Verification items for the finished model (mm, model axes). Round coordinates to 2 decimals unless told otherwise and drop trailing zeros. Loops run counter-clockwise (first coordinate to the right, second up) from the corner with the lowest first, then second, coordinate; pieces in that order, holes last. Notation, with made-up numbers: (86, -15) -> (110, -15) arc R30 ccw to (110, 9) -> close; hole circle Ø7 at (7.5, -3). An arc over 180 degrees is marked (long way). Use a Markdown table: item, result. Add a question column.
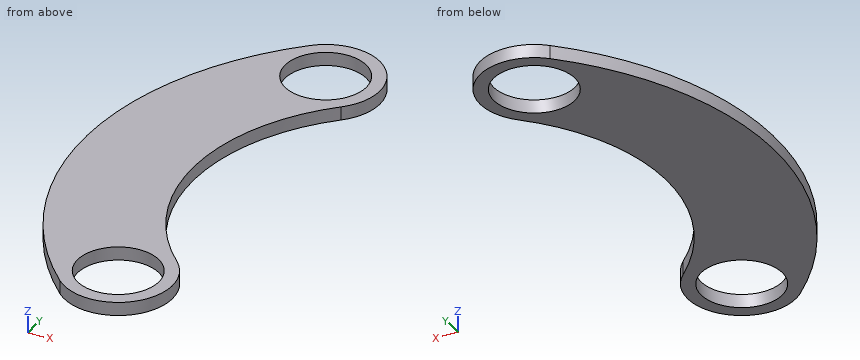
```python
from build123d import *

# Parameters (mm, degrees)
ESQUISSE1_R               = 3
T_LE_DE_BASE_PLI_E1_DEPTH = 1


# Sheet-metal steps are written as plain solids
with BuildPart() as part:
    # Esquisse1 → Tôle de base pliée1 (new body)
    with BuildSketch(Plane.XY):
        with BuildLine():
            ThreePointArc((-57.239284083, -19.336263861), (-64.490656247, -36.242246604), (-57.218655547, -53.139366375))
            ThreePointArc((-57.218655547, -53.139366375), (-51.563834313, -52.987719377), (-51.715481312, -47.332898143))
            ThreePointArc((-51.715481312, -47.332898143), (-56.490657737, -36.237364559), (-51.729027089, -25.136011084))
            ThreePointArc((-51.729027089, -25.136011084), (-51.584281974, -19.481008975), (-57.239284083, -19.336263861))
        make_face()
        with Locations((-54.484155586, -22.236137473)):
            Circle(ESQUISSE1_R, mode=Mode.SUBTRACT)
        with Locations((-54.467068429, -50.236132259)):
            Circle(ESQUISSE1_R, mode=Mode.SUBTRACT)
    extrude(amount=-T_LE_DE_BASE_PLI_E1_DEPTH)


solid = part.part
```
1) Sectioned sample at B-B on y = -49. Enter the section's corners in (x, z).
2) Sectioned sample at D-D on y = -40.5. Enter the section's corners in (x, z), then the cut area to 3 significant figures.
3) Sectioned sample at C-C on z = -0.6. Enter the section's corners in (x, y), then the cut area to 3 significant figures.
4) Go/stop test with a flat-tipped pin: pin 1 (5.5 mm diameter, centred on x = -54.48, y = -22.24, fed in from -Z). Record where the tip stops, or that it passes through.
5) Thickness scan on line 1 (Y direction, x = -54.5, z = -0.9); line 2 (Y direction, x = -52.5, z = -0.8); line 3 (Y direction, x = -51, z = -0.7). Record the ranges inside material, lowest first.
6) Sectioned sample at A-A on x = -53.75. Enter the section's corners in (y, z), then the cut area to 3 significant figures.
Geometry results:
| question | item | result |
|---|---|---|
| 1 | outline | (-60.68, -1) -> (-57.2, -1) -> (-57.2, 0) -> (-60.68, 0) -> close; (-51.73, -1) -> (-50.66, -1) -> (-50.66, 0) -> (-51.73, 0) -> close |
| 2 | outline | (-64.1, -1) -> (-55.88, -1) -> (-55.88, 0) -> (-64.1, 0) -> close |
| 2 | area | 8.21 mm^2 |
| 3 | outline | (-57.24, -19.34) arc R23.3 ccw to (-57.22, -53.14) arc R4 ccw to (-51.72, -47.33) arc R15.3 cw to (-51.73, -25.14) arc R4 ccw to start; hole circle Ø6 at (-54.48, -22.24); hole circle Ø6 at (-54.47, -50.24) |
| 3 | area | 244 mm^2 |
| 4 | pin 1 | through |
| 5 | line 1 | -54.24 to -53.24, -47.24 to -43.77, -28.68 to -25.24, -19.24 to -18.24 |
| 5 | line 2 | -53.72 to -52.5, -47.97 to -46.53, -25.92 to -24.49, -19.99 to -18.76 |
| 5 | line 3 | -52.23 to -48.24, -24.2 to -20.27 |
| 6 | outline | (-54.17, -1) -> (-53.15, -1) -> (-53.15, 0) -> (-54.17, 0) -> close; (-47.32, -1) -> (-44.97, -1) -> (-44.97, 0) -> (-47.32, 0) -> close; (-27.49, -1) -> (-25.14, -1) -> (-25.14, 0) -> (-27.49, 0) -> close; (-19.33, -1) -> (-18.3, -1) -> (-18.3, 0) -> (-19.33, 0) -> close |
| 6 | area | 6.75 mm^2 |
